```python
from build123d import *

# Parameters (mm, degrees)
EXTRUDE_1_DEPTH     = 41
FILLET_4_R          = 8
SKETCH_2_R          = 6
CUT_EXTRUDE_1_DEPTH = 115.5
SKETCH_3_W          = 16
SKETCH_3_H          = 36
CUT_EXTRUDE_2_DEPTH = 400
SKETCH_4_W          = 70
SKETCH_4_H          = 36
CUT_EXTRUDE_3_DEPTH = 12
FILLET_5_R          = 12
FILLET_6_R          = 12
SKETCH_5_R          = 4
SKETCH_5_R_2        = 5
EXTRUDE_2_DEPTH     = 19
SKETCH_6_W          = 3
SKETCH_6_H          = 63
SKETCH_6_W_2        = 24
CUT_EXTRUDE_4_DEPTH = 68


with BuildPart() as part:
    # Эскиз1 → Бобышка-Вытянуть1 (new body)
    with BuildSketch(Plane(origin=(0, 0, 0), x_dir=(1, 0, 0), z_dir=(0, 1, 0))):
        Polygon((0, 0), (14, 0), (20, -60), (20, -490), (0, -490), (0, -140), (-165, -140), (-165, -490), (-185, -490), (-185, -60), (-179, 0), (-165, 0), (-165, -115), (0, -115), align=None)
    extrude(amount=EXTRUDE_1_DEPTH)

    # Скругление4
    fillet_4_edges = [part.edges().sort_by_distance(p)[0] for p in [
        (-82.5, 0, 140),
        (-82.5, 0, 115),
        (-82.5, 41, 140),
        (-82.5, 41, 115),
    ]]
    fillet(fillet_4_edges, radius=FILLET_4_R)

    # Эскиз2 → Вырез-Вытянуть1 (cut, symmetric)
    with BuildSketch(Plane(origin=(-82.5, 0, 0), x_dir=(0, 0, -1), z_dir=(1, 0, 0))):
        with Locations((-17, 20.5)):
            Circle(SKETCH_2_R)
        with BuildLine():
            Line((-462, 26.5), (-441, 26.5))
            ThreePointArc((-441, 26.5), (-435, 20.5), (-441, 14.5))
            Line((-441, 14.5), (-462, 14.5))
            ThreePointArc((-462, 14.5), (-468, 20.5), (-462, 26.5))
        make_face()
    extrude(amount=CUT_EXTRUDE_1_DEPTH, both=True, mode=Mode.SUBTRACT)

    # Эскиз3 → Вырез-Вытянуть2 (cut)
    with BuildSketch(Plane.XY.offset(490)):
        with Locations((10, 20.5)):
            Rectangle(SKETCH_3_W, SKETCH_3_H)
        with Locations((-175, 20.5)):
            Rectangle(SKETCH_3_W, SKETCH_3_H)
    extrude(amount=-CUT_EXTRUDE_2_DEPTH, mode=Mode.SUBTRACT)

    # Эскиз4 → Вырез-Вытянуть3 (cut)
    with BuildSketch(Plane.ZY.offset(185)):
        with Locations((20, 20.5)):
            Rectangle(SKETCH_4_W, SKETCH_4_H)
    cut_extrude_3 = extrude(amount=-CUT_EXTRUDE_3_DEPTH, mode=Mode.SUBTRACT)

    # Зеркальное отражение1: Вырез-Вытянуть3 across plane
    add(cut_extrude_3.mirror(Plane(origin=(-82.5, 0, 0), x_dir=(0, 0, 1), z_dir=(1, 0, 0))), mode=Mode.SUBTRACT)

    # Скругление5
    # the kernel refuses this fillet: 12 mm, written as the material it takes off along each edge
    with BuildSketch(Plane(origin=(20, -1.496268634, 60), x_dir=(-0.0995037190210001, 0, -0.995037190209989), z_dir=(0, 1, 0))) as fillet_5_piece_1:
        with BuildLine():
            CenterArc((FILLET_5_R * 0.0498756211209, FILLET_5_R), FILLET_5_R, 264.289406863, 5.710593137)
            Line((-FILLET_5_R * 0.0496280979001, FILLET_5_R * 0.00496280979001), (0, 0))
            Line((0, 0), (FILLET_5_R * 0.0498756211209, 0))
        make_face()
    extrude(amount=43.992537267, mode=Mode.SUBTRACT)

    # Скругление6
    # the kernel refuses this fillet: 12 mm, written as the material it takes off along each edge
    with BuildSketch(Plane(origin=(-185, -1.496268634, 60), x_dir=(0.09950371902099304, 0, -0.9950371902099898), z_dir=(0, 1, 0))) as fillet_6_piece_1:
        with BuildLine():
            CenterArc((FILLET_6_R * 0.0498756211209, -FILLET_6_R), FILLET_6_R, 90, 5.710593137)
            Line((-FILLET_6_R * 0.0496280979001, -FILLET_6_R * 0.00496280979001), (0, 0))
            Line((0, 0), (FILLET_6_R * 0.0498756211209, 0))
        make_face()
    extrude(amount=43.992537267, mode=Mode.SUBTRACT)

    # Эскиз5 → Бобышка-Вытянуть2 (add, symmetric)
    with BuildSketch(Plane(origin=(-82.5, 0, 0), x_dir=(0, 0, -1), z_dir=(1, 0, 0))):
        with BuildLine():
            Line((-140, 61.173848335), (-140, -17))
            ThreePointArc((-140, -17), (-128.913133611, -29.858457131), (-114.563089264, -20.784607158))
            Line((-114.563089264, -20.784607158), (-103.54711014, 15.415913355))
            ThreePointArc((-103.54711014, 15.415913355), (-102.693554475, 20.5247626), (-103.180589505, 25.681476162))
            Line((-103.180589505, 25.681476162), (-109.885999017, 55.110773465))
            ThreePointArc((-109.885999017, 55.110773465), (-109.847393001, 59.716977585), (-107.748140134, 63.81719029))
            Line((-107.748140134, 63.81719029), (-94.581616231, 79.272692454))
            ThreePointArc((-94.581616231, 79.272692454), (-96.272692454, 100.418383769), (-117.418383769, 98.727307546))
            Line((-117.418383769, 98.727307546), (-132.836767538, 80.628463428))
            ThreePointArc((-132.836767538, 80.628463428), (-138.152291436, 71.539584533), (-140, 61.173848335))
        make_face()
        with Locations((-127, -17)):
            Circle(SKETCH_5_R, mode=Mode.SUBTRACT)
        with Locations((-106, 89)):
            Circle(SKETCH_5_R_2, mode=Mode.SUBTRACT)
    extrude(amount=EXTRUDE_2_DEPTH, both=True)

    # Эскиз6 → Вырез-Вытянуть4 (cut)
    with BuildSketch(Plane.XY.offset(140)):
        with Locations((-100, 72.5)):
            Rectangle(SKETCH_6_W, SKETCH_6_H)
        Polygon((-101.513854398, -4), (-98.5, 0), (-101.5, 0), align=None)
        Polygon((-94.5, 0), (-70.5, 0), (-67.5, -4), (-67.5, -30), (-97.5, -30), (-97.5, -4), align=None)
        with Locations((-82.5, 72.5)):
            Rectangle(SKETCH_6_W_2, SKETCH_6_H)
        Polygon((-63.486145602, -4), (-63.5, 0), (-66.5, 0), align=None)
        with Locations((-65, 72.5)):
            Rectangle(SKETCH_6_W, SKETCH_6_H)
    extrude(amount=-CUT_EXTRUDE_4_DEPTH, mode=Mode.SUBTRACT)


solid = part.part
```
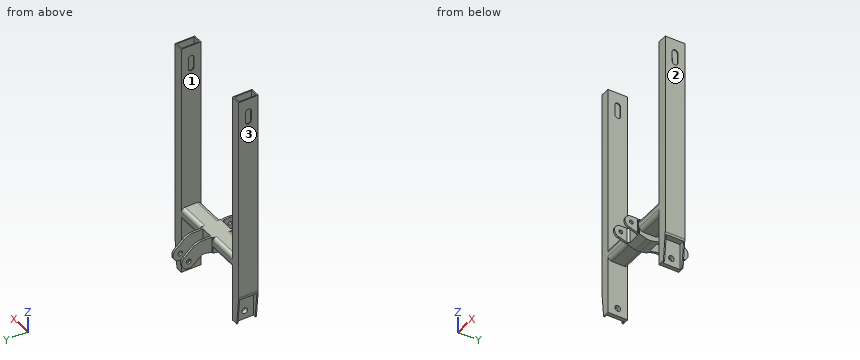
The listing builds one solid part. Answer for the finished solid, in the listing's coordinates (mm). Face numbers are marked on the shaded views. Coordinates: 2 decimals unless noted, no trailing zeros. Write each loop counter-clockwise with the first axis right and the second up, starting at its lowest first coordinate (ties: lowest second). Pieces come first, ordered by that corner, then holes.
Q1. Section C-C, the plane z = 17 is taken. Write down the section's boundary in (x, y), then the cut area to 3 significant figures.
Returned:
outline: (-180.7, 0) - (-165, 0) - (-165, 14.5) - (-173, 14.5) - (-173, 2.5) - (-180.7, 2.5) - close; (-180.7, 38.5) - (-173, 38.5) - (-173, 26.5) - (-165, 26.5) - (-165, 41) - (-180.7, 41) - close; (0, 0) - (15.7, 0) - (15.7, 2.5) - (8, 2.5) - (8, 14.5) - (0, 14.5) - close; (0, 26.5) - (8, 26.5) - (8, 38.5) - (15.7, 38.5) - (15.7, 41) - (0, 41) - close
area: 541 mm2
Q2. Given P1, Ø9, axis at x = 14, z = 29.5, coming from the +Y side; P2, Ø1, axis at x = 1.5, z = 447.5, coming from the -Y side; P3, Ø16, axis at y = 89, z = 106, coming from the +X side, each flat-ended and moving along its own axis, determine where each tip first touches the part or whether it passes through.
Returned:
P1: stops at y = 41
P2: stops at y = 0
P3: stops at x = -66.5
Q3. Section A-A, the plane z = 425 is taken. Write down the section's boundary in (x, y), then the cut area to 3 significant figures.
Returned:
outline: (-185, 0) - (-165, 0) - (-165, 41) - (-185, 41) - close; (0, 0) - (20, 0) - (20, 41) - (0, 41) - close; hole (-183, 2.5) - (-167, 2.5) - (-167, 38.5) - (-183, 38.5) - close; hole (2, 2.5) - (18, 2.5) - (18, 38.5) - (2, 38.5) - close
area: 488 mm2
Q4. Find the intervals of material crossed by line 1 along X through (y, z) = (12.5, 465.5); line 2 along X through (y, z) = (42, 128); line 3 along Y through (x, z) = (-171, 311.5), in increasing order.
Returned:
line 1: x = -185 to -183, -167 to -165, 0 to 2, 18 to 20
line 2: x = -98.5 to -94.5, -70.5 to -66.5
line 3: y = 0 to 2.5, 38.5 to 41
Q5. Section D-D, the plane x = -111 is taken. Write down the section's boundary in (y, z), then the cut area to 3 significant figures.
Returned:
outline: (0, 123) arc R8 ccw to (8, 115) - (33, 115) arc R8 ccw to (41, 123) - (41, 132) arc R8 ccw to (33, 140) - (8, 140) arc R8 ccw to (0, 132) - close
area: 970 mm2
Q6. Section B-B, the plane y = 89 is taken. Write down the section's boundary in (x, z), then the cut area to 3 significant figures.
Returned:
outline: (-98.5, 91) - (-94.5, 91) - (-94.5, 101) - (-98.5, 101) - close; (-98.5, 111) - (-94.5, 111) - (-94.5, 125.71) - (-98.5, 125.71) - close; (-70.5, 91) - (-66.5, 91) - (-66.5, 101) - (-70.5, 101) - close; (-70.5, 111) - (-66.5, 111) - (-66.5, 125.71) - (-70.5, 125.71) - close
area: 198 mm2
Q7. The mould has two halves that part along X. Classify the marked faces 1, 2 and 3: released by +X, released by -X, zero draft, split by the parting line, or undercut.
Returned:
face 1: undercut
face 2: released by +X
face 3: released by -X
